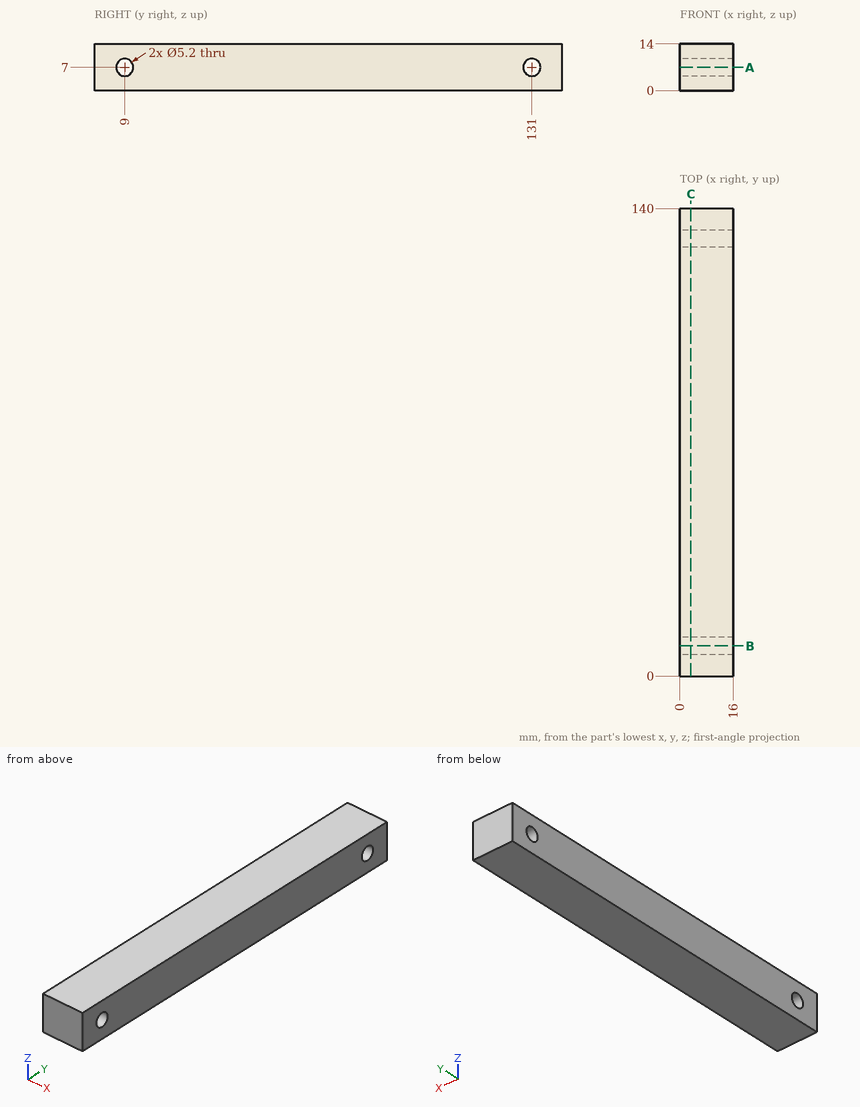
Verification items for this drawing (mm, ordinates from the low corner). Round coordinates to 2 decimals unless told otherwise and drop trailing zeros. Order: outer loops, then holes, each group sorted by start corner. A loop starts at its lowest first (then second) coordinate and runs counter-clockwise, first axis right, second up. Notation, with made-up numbers: (32.25, 24.25) - (52.25, 24.25) arc R20 ccw to (52.25, 43.25) - close; hole circle Ø9 at (7, 7). An arc over 180 degrees is marked (long way). Answer as CSV lines item,"result". Start each with the question number.
1) Section check C-C (x = 3.25). Record the cut outline in (y, z).
2) Depth check by flat-ended pin: pin 1 (4 mm diameter, centred on y = 9, z = 7, fed in from +X). Enter the tip coordinate at first touch or a pass-through.
3) Section check B-B (y = 9). Record the cut outline in (x, z).
4) Scan lines: probe 1 along Y at (x, z) = (13.5, 6.75); probe 2 along Z at (x, y) = (5.25, 131); probe 3 along Y at (x, z) = (11.5, 6). Record each from-to range of solid material in increasing order.
5) Section check A-A (z = 7). Record the cut outline in (x, y), then the cut area to 3 significant figures.
Determined:
1,outline,"(0, 0) - (140, 0) - (140, 14) - (0, 14) - close; hole circle Ø5.2 at (9, 7); hole circle Ø5.2 at (131, 7)"
2,pin 1,"through"
3,outline,"(0, 0) - (16, 0) - (16, 4.4) - (0, 4.4) - close; (0, 9.6) - (16, 9.6) - (16, 14) - (0, 14) - close"
4,probe 1,"0 to 6.41, 11.59 to 128.41, 133.59 to 140"
4,probe 2,"0 to 4.4, 9.6 to 14"
4,probe 3,"0 to 6.6, 11.4 to 128.6, 133.4 to 140"
5,outline,"(0, 0) - (16, 0) - (16, 6.4) - (0, 6.4) - close; (0, 11.6) - (16, 11.6) - (16, 128.4) - (0, 128.4) - close; (0, 133.6) - (16, 133.6) - (16, 140) - (0, 140) - close"
5,area,"2,070 mm^2"
